Design review of the part built by this model. Coordinates are the model's own, in mm. A direction names the side the tool comes from. Coordinates: 2 decimals unless noted, no trailing zeros. Loops run counter-clockwise (first coordinate to the right, second up) from the corner with the lowest first, then second, coordinate; pieces in that order, holes last. Notation, with made-up numbers: M 86,77.25 L 102,77.25 A12 ccw 102,96.25 Z; hole C -20,51.25 d10. An arc over 180 degrees is marked long. Answer as a JSON object with one key per item and string values. Group by question number.
1. Consider section B-B (z = 20.4). State the section outline as (x, y) points.
2. Insertion check: pin 1 (1.5 mm diameter, centred on y = 39.5, z = 21, fed in from +X); pin 2 (1 mm diameter, centred on x = -57.5, z = 20, fed in from +Y); pin 3 (0.6 mm diameter, centred on x = -59, z = 20.5, fed in from -Y). Each pin has a flat end and moves straight along its axis. Give the tip position at first contact, or say it passes through.
3. Consider section C-C (x = -37). State the section outline as (y, z) points.
4. Consider section A-A (y = 35). State the section outline as (x, z) points, then the cut area to 3 significant figures.
5. Machinability: for faces 1 (the flat face through (-48.43, 35, 21)), 2 (the flat face through (-52.389, -2, 20)), 3 (the flat face through (-18.43, 44, 20)), 4 (the flat face through (-18.43, -2, 20)), which of the approach directions +Z, -Z, +X, -X, +Y, -Y give a long, thin tool a straight path to every point of the face, cutting with its end or side? Answer none if there is none.
6. To check wall thickness, follow probe 1 along X at (y, z) = (36, 21.15); probe 2 along Y at (x, z) = (-30, 21.4); probe 3 along Y at (x, z) = (-14, 20). State the ranges of each line that lie inside material, in increasing order.
7. Draft analysis for pull direction X (two halves, no side actions). For faces 5 (the flat face through (-36, 24.997, 21)), 6 (the flat face through (-54.4, 2, 19.2)), 7 (the flat face through (-16.474, 39.951, 21.746)), state which applies: +X half, -X half, draft (parallel to the pull), parting line (faces both ways), or undercut.
Autodesk Inventor part; units mm, degrees
ref_plane "Work Plane1" through (-56.3599, 0, 22) normal (0, 0, -1) x (-1, 0, 0)
ref_plane "YZ Plane" through (0, 0, 0) normal (1, 0, 0) x (0, 1, 0)
ref_plane "XZ Plane" through (0, 0, 0) normal (0, 1, 0) x (-1, 0, 0)
ref_plane "Work Plane1" through (-56.3599, 0, 22) normal (0, 0, -1) x (-1, 0, 0)
sketch "Sketch1" plane through (-56.3599, 0, 22) normal (0, 0, -1) x (-1, 0, 0)
  line L0 (-4.0299, -0.3538) -> (-2.2322, 1.4439) construction
  arc A0 (-1.4439, 2.2322) -> (-2.2322, 1.4439) centre (-0.9299, 0.9299) ccw construction
  line L1 (-1.4439, 2.2322) -> (0.3538, 4.0299) construction
  line L2 (-37.8299, 42.8299) -> (-37.8299, 37.8299) construction
  line L3 (-37.8299, 37.8299) -> (-42.9208, 37.8299) construction
  line L4 (-37.8299, 42.2137) -> (-37.8299, 45.8299) construction
  line L5 (-37.8299, 45.8299) -> (-4.0299, 45.8299) construction
  line L6 (-4.0299, 45.8299) -> (-4.0299, 42.2137) construction
  line L7 (-4.0299, 4.0299) -> (0.3538, 4.0299)
  circle A1 centre (-20.9299, 20.9299) radius 17.5
  line L8 (-20.9299, 58.9723) -> (17.1124, 20.9299) construction
  line L9 (17.1124, 20.9299) -> (-20.9299, -17.1124) construction
  line L10 (-20.9299, -17.1124) -> (-58.9723, 20.9299) construction
  line L11 (-58.9723, 20.9299) -> (-20.9299, 58.9723) construction
  line L12 (-20.9299, 58.9723) -> (-20.9299, -17.1124) construction
  line L13 (17.1124, 20.9299) -> (-58.9723, 20.9299) construction
  line L14 (-20.9299, 58.9723) -> (32.8701, 58.9723) construction
  line L15 (-43.4299, 43.4299) -> (1.5701, 43.4299) construction
  line L16 (1.5701, 43.4299) -> (1.5701, -1.5701) construction
  line L17 (1.5701, -1.5701) -> (-43.4299, -1.5701) construction
  line L18 (-43.4299, -1.5701) -> (-43.4299, 43.4299) construction
  line L19 (-43.4299, 43.4299) -> (1.5701, -1.5701) construction
  line L20 (1.5701, 43.4299) -> (-43.4299, -1.5701) construction
  line L21 (-43.4299, 5.3876) -> (-43.4299, 36.4723)
  line L22 (-43.4299, 36.4723) -> (-36.4723, 43.4299)
  line L23 (-36.4723, 43.4299) -> (-5.3876, 43.4299)
  line L24 (-5.3876, 43.4299) -> (1.5701, 36.4723)
  line L25 (1.5701, 36.4723) -> (1.5701, 5.3876)
  line L26 (1.5701, 5.3876) -> (-5.3876, -1.5701)
  line L27 (-5.3876, -1.5701) -> (-36.4723, -1.5701)
  line L28 (-36.4723, -1.5701) -> (-43.4299, 5.3876)
  line L29 (-4.0299, 42.2137) -> (-37.8299, 42.2137)
  line L30 (-4.0299, -0.3538) -> (-4.0299, 4.0299)
  circle A2 centre (-20.9299, 20.9299) radius 1.5
  line L31 (-10.9299, 10.9299) -> (-30.9299, 10.9299) construction
  line L32 (-30.9299, 10.9299) -> (-30.9299, 30.9299) construction
  line L33 (-30.9299, 30.9299) -> (-10.9299, 30.9299) construction
  line L34 (-10.9299, 30.9299) -> (-10.9299, 10.9299) construction
  line L35 (-10.9299, 10.9299) -> (-30.9299, 30.9299) construction
  line L36 (-30.9299, 10.9299) -> (-10.9299, 30.9299) construction
  circle A3 centre (-30.9299, 30.9299) radius 1.4
  circle A4 centre (-30.9299, 10.9299) radius 1.4
  circle A5 centre (-10.9299, 10.9299) radius 1.4
  line L37 (-45.8299, 37.8299) -> (-42.0723, 37.8299) construction
  line L38 (-42.1723, 37.7299) -> (-45.8299, 37.7299)
  line L39 (-45.8299, 37.7299) -> (-45.8299, 4.1299)
  line L40 (-45.8299, 4.1299) -> (-42.1723, 4.1299)
  line L41 (-42.1723, 4.1299) -> (-42.1723, 37.7299)
  line L42 (-45.8299, 4.0299) -> (-42.0723, 4.0299) construction
  line L43 (-45.8299, 37.8299) -> (-42.0723, 37.8299)
  line L44 (-37.7299, 45.8299) -> (-4.1299, 45.8299)
  line L45 (-4.1299, 45.8299) -> (-4.1299, 42.1723)
  line L46 (-4.1299, 42.1723) -> (-37.7299, 42.1723)
  line L47 (-37.7299, 42.1723) -> (-37.7299, 45.8299)
  line L48 (0.4701, 37.8299) -> (0.4701, 4.0299) construction
  line L49 (0.4701, 4.0299) -> (3.9701, 4.0299) construction
  line L50 (3.9701, 37.8299) -> (3.9701, 4.0299) construction
  line L51 (0.4701, 37.8299) -> (3.9701, 37.8299) construction
  line L52 (-45.8299, -3.9701) -> (-4.0299, -3.9701) construction
  line L53 (0.3124, 37.7299) -> (3.9701, 37.7299)
  line L54 (3.9701, 37.7299) -> (3.9701, 4.1299)
  line L55 (3.9701, 4.1299) -> (0.3124, 4.1299)
  line L56 (0.3124, 4.1299) -> (0.3124, 37.7299)
  line L57 (-4.1713, -0.3538) -> (-37.7299, -0.3538)
  line L58 (-37.7299, -0.3538) -> (-37.7299, -3.9701)
  line L59 (-37.7299, -3.9701) -> (-4.1713, -3.9701)
  line L60 (-4.1713, -3.9701) -> (-4.1713, -0.3538)
  point P0 (-37.8299, 4.0299)
  dimension "d18" = 53.8
  dimension "d19" = 45
  dimension "d20" = 53.8
  dimension "d21" = 45
  dimension "d22" = 45
  dimension "d30" = 20
  dimension "d31" = 20
  dimension "d32" = 2.8
  dimension "d33" = 2.8
  dimension "d34" = 2.8
  dimension "d35" = 3
  dimension "d36" = 0.1
  dimension "d37" = 0.1
  dimension "d38" = 0.1
  dimension "d39" = 0.1
extrude "Extrusion1" add sketch "Sketch1" along normal blind 3 contours L30 L26 L57 L28 L41 L22 L46 L24 L56 L7 | L7 L26 L30 | L56 L24 L25 L26 | L26 L25 L24 L53 L54 L55 | L60 L59 L58 L57 L28 L27 L26 | L26 L27 L28 L57 | L46 L22 L29 L24 | L24 L29 L45 | L40 L39 L38 L22 L21 L28 | L28 L21 L22 L41 | L29 L22 L23 L24 | L24 L23 L22 L29 L47 L44 L45 | L47 L29 L22 | A1 | A2 | A3 | A4 | A5
sketch "Skizze4" plane through (-56.3599, 0, 19) normal (0, 0, -1) x (-1, 0, 0)
  line L0 (-37.7299, 42.1723) -> (-42.1723, 37.7299)
  line L1 (-42.1723, 37.7299) -> (-45.8299, 37.7299)
  line L2 (-45.8299, 37.7299) -> (-45.8299, 4.1299) construction
  line L3 (-45.8299, 4.1299) -> (-42.1723, 4.1299)
  line L4 (-42.1723, 4.1299) -> (-37.6885, -0.3538)
  line L5 (-37.6885, -0.3538) -> (-37.7299, -0.3538)
  line L6 (-37.7299, -0.3538) -> (-37.7299, -3.9701)
  line L7 (-37.7299, -3.9701) -> (-4.1713, -3.9701) construction
  line L8 (-4.1713, -3.9701) -> (-4.1713, -0.3538)
  line L9 (-4.1713, -0.3538) -> (0.3124, 4.1299)
  line L10 (0.3124, 4.1299) -> (3.9701, 4.1299)
  line L11 (3.9701, 4.1299) -> (3.9701, 37.7299) construction
  line L12 (3.9701, 37.7299) -> (0.3124, 37.7299)
  line L13 (0.3124, 37.7299) -> (-4.1299, 42.1723)
  line L14 (-4.1299, 42.1723) -> (-4.1299, 45.8299)
  line L15 (-4.1299, 45.8299) -> (-37.7299, 45.8299) construction
  line L16 (-37.7299, 45.8299) -> (-37.7299, 42.1723)
  line L17 (-37.9299, 46.0299) -> (-3.9299, 46.0299) construction
  line L18 (-3.9299, 46.0299) -> (-3.9299, 42.2551)
  line L19 (-3.9299, 42.2551) -> (0.3953, 37.9299)
  line L20 (0.3953, 37.9299) -> (4.1701, 37.9299)
  line L21 (4.1701, 37.9299) -> (4.1701, 3.9299) construction
  line L22 (4.1701, 3.9299) -> (0.3953, 3.9299)
  line L23 (0.3953, 3.9299) -> (-3.9713, -0.4367)
  line L24 (-3.9713, -0.4367) -> (-3.9713, -4.1701)
  line L25 (-3.9713, -4.1701) -> (-37.9299, -4.1701) construction
  line L26 (-37.9299, -4.1701) -> (-37.9299, -0.3953)
  line L27 (-37.9299, -0.3953) -> (-42.2551, 3.9299)
  line L28 (-42.2551, 3.9299) -> (-46.0299, 3.9299)
  line L29 (-46.0299, 3.9299) -> (-46.0299, 37.9299) construction
  line L30 (-46.0299, 37.9299) -> (-42.2551, 37.9299)
  line L31 (-42.2551, 37.9299) -> (-37.9299, 42.2551)
  line L32 (-37.9299, 42.2551) -> (-37.9299, 46.0299)
  line L33 (-45.8299, 37.7299) -> (-45.8299, 37.9299)
  line L34 (-4.1299, 45.8299) -> (-37.7299, 45.8299)
  line L35 (-37.7299, 45.8299) -> (-37.9299, 45.8299)
  line L36 (-4.1299, 45.8299) -> (-3.9299, 45.8299)
  line L37 (3.9701, 37.7299) -> (3.9701, 37.9299)
  line L38 (3.9701, 4.1299) -> (3.9701, 37.7299)
  line L39 (3.9701, 4.1299) -> (3.9701, 3.9299)
  line L40 (-4.1713, -3.9701) -> (-3.9713, -3.9701)
  line L41 (-37.7299, -3.9701) -> (-37.9299, -3.9701)
  line L42 (-45.8299, 4.1299) -> (-45.8299, 3.9299)
  point P0 (-56.3599, 0)
  dimension "d40" = 0.2
extrude "IM_offset" add sketch "Skizze4" against normal up to surface (3 mm away)
ref_plane "Arbeitsebene5" through (-35.4299, 3.9299, 22) normal (-1, 0, 0) x (0, 0, 1)
ref_plane "Arbeitsebene6" through (-18.4299, 20.9299, 22) normal (0, 1, 0) x (-1, 0, 0)
chamfer "Fase2" distance 0.5 angle 45 32 edges at (-35.4299, 45.8299, 22) (-18.4299, 44.0425, 22) (-16.2673, 40.0925, 22) (-12.3173, 37.9299, 22) (-10.5299, 20.9299, 22) (-12.3173, 3.9299, 22) (-16.2673, 1.7673, 22) (-18.4299, -2.1827, 22) (-35.4092, -3.9701, 22) (-52.3885, -2.2034, 22) (-54.5718, 1.7466, 22) (-58.5425, 3.9299, 22) (-60.3299, 20.9299, 22) (-58.5425, 37.9299, 22) (-54.5925, 40.0925, 22) (-54.5718, 1.7466, 19) (-58.5425, 3.9299, 19) (-60.3299, 20.9299, 19) (-52.3885, -2.2034, 19) (-35.4092, -3.9701, 19) (-18.4299, -2.1827, 19) (-16.2673, 1.7673, 19) (-12.3173, 3.9299, 19) (-10.5299, 20.9299, 19) (-12.3173, 37.9299, 19) (-16.2673, 40.0925, 19) (-18.4299, 44.0425, 19) (-35.4299, 45.8299, 19) (-52.4299, 44.0425, 19) (-54.5925, 40.0925, 19) (-58.5425, 37.9299, 19) (-52.4299, 44.0425, 22)
sketch "Skizze33" plane through (-56.3599, 0, 22) normal (0, 0, 1) x (1, 0, 0)
  line L0 (35.9299, 55.1649) -> (35.9299, -0.2255)
  line L1 (35.9299, 55.1649) -> (20.9299, 55.1649)
  line L2 (20.9299, 55.1649) -> (20.9299, 47.7466)
  line L3 (33.9299, 47.7466) -> (20.9299, 47.7466)
  line L4 (33.9299, 24.9969) -> (33.9299, 47.7466)
  line L5 (20.9299, 24.9969) -> (33.9299, 24.9969)
  line L6 (20.9299, 24.9969) -> (20.9299, 20.7437)
  line L7 (22.9299, 20.7437) -> (20.9299, 20.7437)
  line L8 (22.9299, 17.3807) -> (22.9299, 20.7437)
  line L9 (20.9299, 17.3807) -> (22.9299, 17.3807)
  line L10 (20.9299, 17.3807) -> (20.9299, -0.2255)
  line L11 (35.9299, -0.2255) -> (20.9299, -0.2255)
  line L12 (20.9299, 24.9969) -> (33.9299, 24.9969)
  line L13 (33.9299, 24.9969) -> (33.9299, 47.7466)
  line L14 (33.9299, 47.7466) -> (20.9299, 47.7466)
  line L15 (20.9299, 47.7466) -> (20.9299, 24.9969)
  line L16 (20.9299, 24.9969) -> (7.9299, 24.9969)
  line L17 (7.9299, 24.9969) -> (7.9299, 47.7466)
  line L18 (7.9299, 47.7466) -> (20.9299, 47.7466)
  line L19 (20.9299, 47.7466) -> (20.9299, 24.9969)
  point P0 (56.3599, 0)
  dimension "d189" = 13
extrude "Extrusion28" cut sketch "Skizze33" against normal blind 3 contours L3 L4 L5 L15 | L15 L16 L17 L18
properties part number "20_Cube_Insert_Filter_25mm"
Findings below:
{
 "1": {"outline": "M -60.33,3.93 L -56.76,3.93 L -52.39,-0.44 L -52.39,-3.97 L -18.43,-3.97 L -18.43,-0.4 L -14.1,3.93 L -10.53,3.93 L -10.53,37.93 L -14.1,37.93 L -18.43,42.26 L -18.43,45.83 L -22.43,45.83 L -22.43,25 L -48.43,25 L -48.43,45.83 L -52.43,45.83 L -52.43,42.26 L -56.76,37.93 L -60.33,37.93 Z"},
 "2": {"pin 1": "stops at x = -14.92", "pin 2": "stops at y = 37.93", "pin 3": "stops at y = 3.93"},
 "3": {"outline": "M -3.97,19.5 L -3.47,19 L 25,19 L 25,22 L -3.47,22 L -3.97,21.5 Z"},
 "4": {"outline": "M -60.33,19.5 L -59.83,19 L -48.43,19 L -48.43,22 L -59.83,22 L -60.33,21.5 Z; M -22.43,19 L -11.03,19 L -10.53,19.5 L -10.53,21.5 L -11.03,22 L -22.43,22 Z", "area": "70.9 mm^2"},
 "5": {"face 1": "+Z, -Z, +Y", "face 2": "+Z, -Z, -X, -Y", "face 3": "+Z, -Z, +X, +Y", "face 4": "+Z, -Z, +X, -Y"},
 "6": {"probe 1": "x = -60.33 to -48.43, -22.43 to -10.53", "probe 2": "y = -3.97 to 25", "probe 3": "y = 3.93 to 37.93"},
 "7": {"face 5": "undercut", "face 6": "-X half", "face 7": "+X half"}
}
